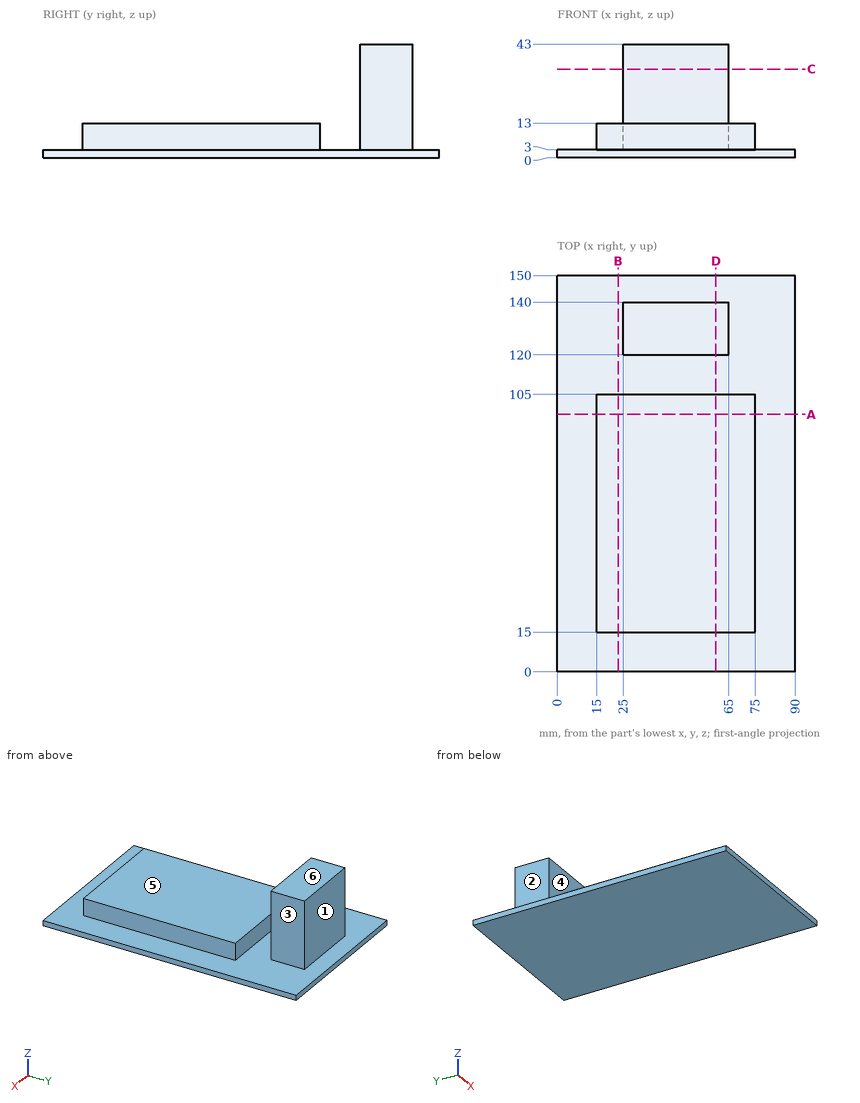
Here's the drawing with two shaded views (mm, measured from the low corner). I have some questions. A direction names the side the tool comes from. Coordinates: 2 decimals unless noted, no trailing zeros. Order: outer loops, then holes, each group sorted by start corner. A loop starts at its lowest first (then second) coordinate and runs counter-clockwise, first axis right, second up. Notation, with made-up numbers: (15.25, 60) - (59.25, 60) arc R17 ccw to (59.25, 91) - close; hole circle Ø3 at (8.5, -36.75). An arc over 180 degrees is marked (long way). Use CSV: the item, a comma, the result in double quotes. Start each with the question number.
1. Please list where these lines run through material, in increasing order: line 1 (Y direction, x = 56, z = 11); line 2 (Z direction, x = 35, y = 54.5); line 3 (X direction, y = 124, z = 28). Write a range as from..to.
2. Suppose I cut it at A-A on y = 97.5. List the corners of the cut face in (x, z) for me, then the cut area to 3 significant figures.
3. Suppose I cut it at C-C on z = 33.5. List the corners of the cut face in (x, y) for me.
4. I'm going to push flat-ended pins straight in: pin 1 (3 mm diameter, centred on x = 47, z = 8.5, fed in from +Y); pin 2 (20 mm diameter, centred on x = 53.5, z = 14, fed in from -Y); pin 3 (10 mm diameter, centred on y = 130.5, z = 33, fed in from +X). Where does each tip first touch, or does it pass through?
5. If we mould it in two halves opening along X, with no side actions, what happens to the marked faces 1, 2 and 3? For each: +X half, -X half, draft (parallel to the pull), parting line (faces both ways), or undercut.
6. Suppose I cut it at D-D on x = 60. List the corners of the cut face in (y, z) for me, then the cut area to 3 significant figures.
7. For the marked faces 4, 5 and 6, which set-ups out of +Z, -Z, +X, -X, +Y, -Y let a thin tool reach every point of the face, with its end or its side?
8. Suppose I cut it at B-B on x = 23. List the corners of the cut face in (y, z) for me, then the cut area to 3 significant figures.
Output:
1,line 1,"y = 15..105, 120..140"
1,line 2,"z = 0..13"
1,line 3,"x = 25..65"
2,outline,"(0, 0) - (90, 0) - (90, 3) - (75, 3) - (75, 13) - (15, 13) - (15, 3) - (0, 3) - close"
2,area,"870 mm2"
3,outline,"(25, 120) - (65, 120) - (65, 140) - (25, 140) - close"
4,pin 1,"stops at y = 140"
4,pin 2,"stops at y = 15"
4,pin 3,"stops at x = 65"
5,face 1,"draft"
5,face 2,"-X half"
5,face 3,"+X half"
6,outline,"(0, 0) - (150, 0) - (150, 3) - (140, 3) - (140, 43) - (120, 43) - (120, 3) - (105, 3) - (105, 13) - (15, 13) - (15, 3) - (0, 3) - close"
6,area,"2,150 mm2"
7,face 4,"+Z, +X, -X"
7,face 5,"+Z, +X, -X, -Y"
7,face 6,"+Z, +X, -X, +Y, -Y"
8,outline,"(0, 0) - (150, 0) - (150, 3) - (105, 3) - (105, 13) - (15, 13) - (15, 3) - (0, 3) - close"
8,area,"1,350 mm2"
